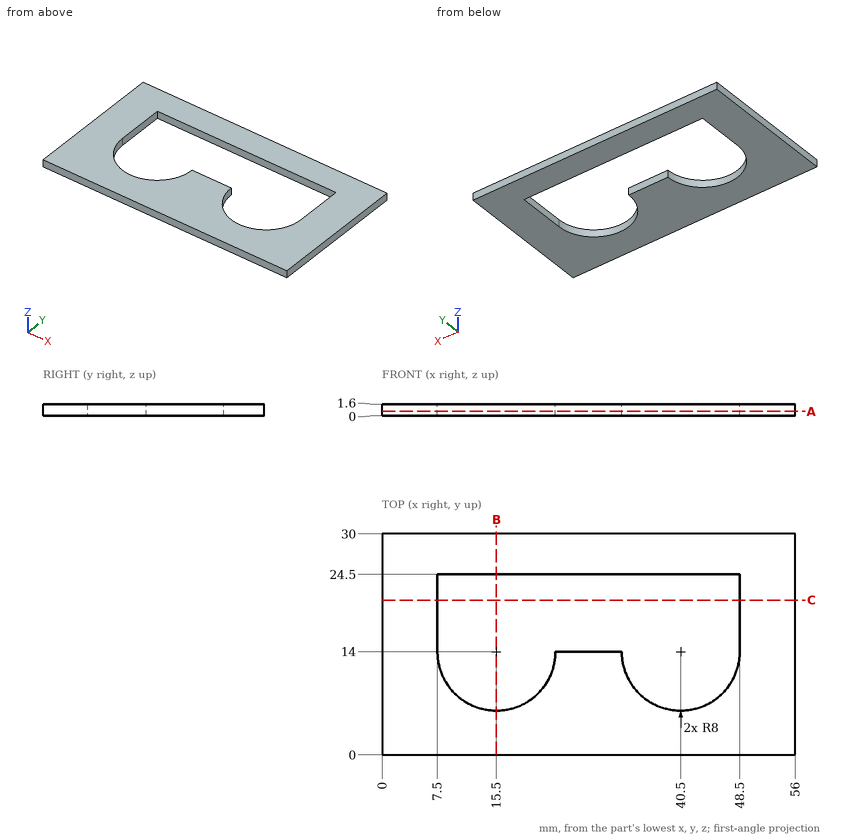
Part print with two shaded views. Sizes in mm from the minimum x, y, z corner. Round coordinates to 2 decimals unless told otherwise and drop trailing zeros. Order: outer loops, then holes, each group sorted by start corner. A loop starts at its lowest first (then second) coordinate and runs counter-clockwise, first axis right, second up. Notation, with made-up numbers: M 67.25,-28 L 100.25,-28 A30 ccw 100.25,3 Z; hole C 44.5,22 d6. An arc over 180 degrees is marked long. Answer in a Markdown table with one row per item. Add a question column.
Q1. Pin check, flat tip, straight feed: pin 1 (12 mm diameter, centred on x = 46.5, y = 11, fed in from -Z). Stop position of the tip, or through.
Q2. Cut at C-C on y = 21. Give the cut face in (x, z).
Q3. Cut at B-B on x = 15.5. Give the cut face in (y, z).
Q4. Cut at A-A on z = 0.6. Give the cut face in (x, y), and give its area (3 significant figures).
Q5. Wall check: L1, parallel to X at y = 20, z = 0.65; L2, parallel to Y at x = 25.5, z = 0.75; L3, parallel to X at y = 11, z = 0.3. Give the ranges that are in metal, low to high. Write a range as from..to.
Established:
| question | item | result |
|---|---|---|
| 1 | pin 1 | stops at z = 0 |
| 2 | outline | M 0,0 L 7.5,0 L 7.5,1.6 L 0,1.6 Z; M 48.5,0 L 56,0 L 56,1.6 L 48.5,1.6 Z |
| 3 | outline | M 0,0 L 6,0 L 6,1.6 L 0,1.6 Z; M 24.5,0 L 30,0 L 30,1.6 L 24.5,1.6 Z |
| 4 | outline | M 0,0 L 56,0 L 56,30 L 0,30 Z; hole M 7.5,14 A8 ccw 23.5,14 L 32.5,14 A8 ccw 48.5,14 L 48.5,24.5 L 7.5,24.5 Z |
| 4 | area | 1,050 mm2 |
| 5 | L1 | x = 0..7.5, 48.5..56 |
| 5 | L2 | y = 0..14, 24.5..30 |
| 5 | L3 | x = 0..8.08, 22.92..33.08, 47.92..56 |
